Autodesk Inventor part; units mm, degrees
ref_plane "YZ Plane" through (0, 0, 0) normal (1, 0, 0) x (0, 1, 0)
ref_plane "XZ Plane" through (0, 0, 0) normal (0, 1, 0) x (-1, 0, 0)
ref_plane "XY Plane" through (0, 0, 0) normal (0, 0, 1) x (1, 0, 0)
sketch "Sketch1" plane through (0, 0, 0) normal (1, 0, 0) x (0, 1, 0)
  line L0 (0, 0) -> (0, -30)
  line L1 (13.5, 0) -> (30, 0) construction
  line L2 (0, -30) -> (85, -30)
  line L3 (13.5, 0) -> (85, 0)
  line L4 (85, 0) -> (85, -30)
  line L5 (0, 0) -> (0, 10.5)
  line L6 (13.5, 0) -> (14, 0) construction
  line L7 (0, 10.5) -> (8.5, 10.5)
  line L8 (8.5, 10.5) -> (8.5, 30.5)
  line L9 (8.5, 30.5) -> (13.5, 30.5)
  line L10 (13.5, 30.5) -> (13.5, 0)
  point P0 (0, -15)
  dimension "d0" = 30
  dimension "d2" = 85
  dimension "d4" = 10.5
  dimension "d6" = 8.5
  dimension "d7" = 20
  dimension "d8" = 5
  dimension "d47" = 30
extrude "Extrusion1" add sketch "Sketch1" along normal blind 50
sketch "Sketch2" plane through (0, 85, 0) normal (0, 1, 0) x (1, 0, 0)
  line L0 (4.5, 4.5) -> (4.5, 25.5)
  line L1 (4.5, 4.5) -> (25.5, 4.5) construction
  line L2 (4.5, 25.5) -> (45.5, 25.5)
  line L3 (45.5, 25.5) -> (45.5, 4.5)
  line L4 (45.5, 4.5) -> (4.5, 4.5)
  line L5 (50, 30) -> (50, 0)
  point P0 (0, 0)
  dimension "d13" = 21
  dimension "d14" = 90
  dimension "d15" = 41
  dimension "d16" = 90
  dimension "d17" = 21
  dimension "d18" = 90
  dimension "d46" = 4.5
  dimension "d48" = 90
  dimension "d49" = 4.5
extrude "Extrusion2" cut sketch "Sketch2" against normal blind 80
fillet "Fillet1" radius 2 12 edges at (50, 85, -15) (25, 85, 0) (25, 85, -30) (0, 85, -15) (50, 49.25, 0) (50, 42.5, -30) (0, 49.25, 0) (0, 42.5, -30) (0, 13.5, 15.25) (25, 13.5, 30.5) (50, 13.5, 15.25) (25, 13.5, 0)
sketch "Sketch4" plane through (2, 13.5, 2) normal (0, 1, 0) x (1, 0, 0)
  line L0 (-2, -28.5) -> (48, -28.5)
  point P0 (-2, 2)
  point P1 (23, -18.5)
  point P2 (23, -28.5)
  dimension "d37" = 10
hole "Hole1" at (25, 13.5, 20.5) direction (0, -1, 0) diameter 5 end through all countersink diameter 10 countersink angle 77.33
sketch "Sketch6" plane through (50, 0, 0) normal (1, 0, 0) x (0, 0, -1)
  line L0 (-10.5, 0) -> (28, 0)
  point P0 (0, 0)
  point P1 (15, 59)
  point P2 (15, 0)
  dimension "d45" = 59
hole "Hole2" at (50, 59, -15) direction (-1, 0, 0) diameter 5 end through all
chamfer "Chamfer2" distance 2 angle 45 4 edges at (4.5, 85, -15) (25, 85, -25.5) (45.5, 85, -15) (25, 85, -4.5)
fillet "Fillet3" radius 2 4 edges at (3.5, 84, -26.5) (46.5, 84, -26.5) (46.5, 84, -3.5) (3.5, 84, -3.5)
properties part number "flexibler_standfuß_breit_v0.9"
Design review of the part built by this model. Coordinates are the model's own, in mm. A direction names the side the tool comes from. Coordinates: 2 decimals unless noted, no trailing zeros. Loops run counter-clockwise (first coordinate to the right, second up) from the corner with the lowest first, then second, coordinate; pieces in that order, holes last. Notation, with made-up numbers: (28, 74.5) - (47, 74.5) arc R20 cw to (47, 93.5) - close; hole circle Ø8 at (83, -18). An arc over 180 degrees is marked (long way). Use CSV: the item, a comma, the result in double quotes. Start each with the question number.
1) The part is to be moulded in two halves that separate along Z. For faces 6 (the flat face through (0, 41, -11)), 7 (the cylindrical face through (25.32, 84.4, -29.43)), 8 (the cylindrical face through (47.72, 57.31, -13.16)), 9 (the cylindrical face through (23, 9, 19)), say which applies: +Z half, -Z half, draft (parallel to the pull), parting line (faces both ways), or undercut.
2) Consider section D-D on z = 20.5. Write out the cut boundary in (x, y), then the cut area to 3 significant figures.
3) Consider section C-C on x = 25. Write out the cut boundary in (y, z).
4) Consider section B-B on z = -15. Write out the cut boundary in (x, y), then the cut area to 3 significant figures.
5) Tool access review of faces 1 (the flat face through (25, 0, -10)), 2 (the cylindrical face through (3.99, 83.88, -25.99)), 3 (the flat face through (25, 4, 10.5)), 4 (the cylindrical face through (0.57, 49.72, -0.6)), 5 (the flat face through (25, 49, 0)): name each direction out of +Z, -Z, +X, -X, +Y, -Y from which nothing blocks a thin tool from reaching the whole face with its end or side.
6) Wall thickness on L1, parallel to Z at x = 25, y = 9.4; L2, parallel to Z at x = 32.5, y = 46; L3, parallel to Y at x = 2, z = -15: over which ranges is each line inside the solid? List them lowest first. Write a range as from..to.
7) For pin 1 Ø3 at (x, z) = (40.5, -20.5) entering from -Y; pin 2 Ø7 at (x, y) = (36, 2.5) entering from +Z; pin 3 Ø8 at (x, z) = (33.5, 18.5) entering from +Y; pin 4 Ø8 at (x, y) = (35.5, 73.5) entering from +Z, all flat-tipped, find the tip position at first contact; note any pin that passes through.
8) Consider section A-A on y = 60.5. Write out the cut boundary in (x, z).
Geometry says:
1,face 6,"draft"
1,face 7,"-Z half"
1,face 8,"undercut"
1,face 9,"undercut"
2,outline,"(0, 8.5) - (22.5, 8.5) - (22.5, 10.38) - (20, 13.5) - (2, 13.5) arc R2 ccw to (0, 11.5) - close; (27.5, 8.5) - (50, 8.5) - (50, 11.5) arc R2 ccw to (48, 13.5) - (30, 13.5) - (27.5, 10.38) - close"
2,area,"215 mm^2"
3,outline,"(0, -30) - (83, -30) arc R2 ccw to (85, -28) - (85, -27.5) - (83, -25.5) - (5, -25.5) - (5, -4.5) - (83, -4.5) - (85, -2.5) - (85, -2) arc R2 ccw to (83, 0) - (15.5, 0) arc R2 cw to (13.5, 2) - (13.5, 15.5) - (10.38, 18) - (8.5, 18) - (8.5, 10.5) - (0, 10.5) - close; (8.5, 23) - (10.38, 23) - (13.5, 25.5) - (13.5, 28.5) arc R2 ccw to (11.5, 30.5) - (8.5, 30.5) - close"
4,outline,"(0, 0) - (50, 0) - (50, 56.5) - (45.5, 56.5) - (45.5, 5) - (4.5, 5) - (4.5, 56.5) - (0, 56.5) - close; (0, 61.5) - (4.5, 61.5) - (4.5, 83) - (2.5, 85) - (2, 85) arc R2 ccw to (0, 83) - close; (45.5, 61.5) - (50, 61.5) - (50, 83) arc R2 ccw to (48, 85) - (47.5, 85) - (45.5, 83) - close"
4,area,"919 mm^2"
5,face 1,"+Z, -Z, +X, -X, -Y"
5,face 2,"+Y"
5,face 3,"+Z, +X, -X, -Y"
5,face 4,"+Z, -X, +Y"
5,face 5,"+Z, +X, -X, +Y"
6,L1,"-30..-25.5, -4.5..18, 23..30.5"
6,L2,"-30..-25.5, -4.5..0"
6,L3,"0..56.5, 61.5..85"
7,pin 1,"y = 0"
7,pin 2,"z = 10.5"
7,pin 3,"y = 13.5"
7,pin 4,"z = 0"
8,outline,"(0, -28) arc R2 ccw to (2, -30) - (48, -30) arc R2 ccw to (50, -28) - (50, -17) - (45.5, -17) - (45.5, -25.5) - (4.5, -25.5) - (4.5, -17) - (0, -17) - close; (0, -13) - (4.5, -13) - (4.5, -4.5) - (45.5, -4.5) - (45.5, -13) - (50, -13) - (50, -2) arc R2 ccw to (48, 0) - (2, 0) arc R2 ccw to (0, -2) - close"
